Autodesk Inventor part; units mm, degrees
ref_plane "YZ Plane" through (0, 0, 0) normal (1, 0, 0) x (0, 1, 0)
ref_plane "XZ Plane" through (0, 0, 0) normal (0, 1, 0) x (-1, 0, 0)
ref_plane "XY Plane" through (0, 0, 0) normal (0, 0, 1) x (1, 0, 0)
sketch "Sketch1" plane through (0, 0, 0) normal (0, 1, 0) x (-1, 0, 0)
  line L0 (7.415, 10.16) -> (-7.415, 10.16)
  line L1 (-7.415, 10.16) -> (-7.415, -10.16)
  line L2 (-7.415, -10.16) -> (7.415, -10.16)
  line L3 (7.415, -10.16) -> (7.415, 10.16)
  point P0 (0, 0)
  dimension "d0" = 20.32
  dimension "d1" = 10.16
  dimension "d2" = 14.83
  dimension "d3" = 7.415
extrude "Extrusion1" add sketch "Sketch1" along normal blind 3.91
sketch "Sketch2" plane through (0, 0, 0) normal (0, 1, 0) x (-1, 0, 0)
  line L0 (6.465, -5.76) -> (7.465, -5.76)
  line L1 (7.465, -5.76) -> (7.465, -4.24)
  line L2 (7.465, -4.24) -> (6.465, -4.24)
  line L3 (6.465, -4.24) -> (6.465, -5.76)
  line L4 (7.415, -10.16) -> (7.415, 10.16)
  line L5 (-7.415, -10.16) -> (7.415, -10.16)
  circle A0 centre (7.465, -5) radius 0.5724
  point P0 (0, 0)
  dimension "d6" = 1
  dimension "d7" = 1.52
  dimension "d8" = 0.05
  dimension "d9" = 4.4
extrude "Extrusion2" cut sketch "Sketch2" along normal blind 1 contours A0 L4 | L4 A0 L1 | L1 A0
pattern_linear "Rectangular Pattern1" count 6 spacing 2.01 along (0, 0, 1) of "Extrusion2"
mirror "Mirror1" about plane through (0, 0, 0) normal (1, 0, 0) of "Extrusion2", "Rectangular Pattern1"
sketch "Sketch3" plane through (0, 0, 0) normal (0, -1, 0) x (1, 0, 0)
  line L0 (3.695, -10.21) -> (-3.695, -10.21)
  line L1 (-3.695, -10.21) -> (-3.695, -9.21)
  line L2 (-3.695, -9.21) -> (3.695, -9.21)
  line L3 (3.695, -9.21) -> (3.695, -10.21)
  line L4 (7.415, -10.16) -> (-7.415, -10.16)
  ellipse E0 centre (0, -10.21) end of major axis (-3.2399, -10.21) minor radius 0.6001
  point P0 (0, 0)
  dimension "d15" = 0.05
  dimension "d16" = 7.39
  dimension "d17" = 3.695
  dimension "d18" = 1
extrude "Extrusion3" cut sketch "Sketch3" against normal blind 1 contours E0 L4 L0 | L0 E0 | E0 L4
mirror "Mirror2" about plane through (0, 0, 0) normal (0, 0, 1) of "Extrusion3"
properties part number "MC_DK1042"
Part model, mm, in its own coordinate system. A direction names the side the tool comes from. Round coordinates to 2 decimals unless told otherwise and drop trailing zeros. Loops run counter-clockwise (first coordinate to the right, second up) from the corner with the lowest first, then second, coordinate; pieces in that order, holes last. Notation, with made-up numbers: (51.5, -4) -> (90.5, -4) arc R18 cw to (90.5, 4) -> close; hole circle Ø8 at (69.5, 21). An arc over 180 degrees is marked (long way). Use CSV: the item, a comma, the result in double quotes. Start each with the question number.
1) Cut at B-B, the plane z = -1.25. Write the cut outline in (x, y) (3 decimals).
2) Cut at A-A, the plane z = 3.25. Write the cut outline in (x, y) (3 decimals).
3) Pull direction Z, two halves, no side cores. Call faces 4 (the cylindrical face through (-6.893, 0.493, -5.012)), 5 (the flat face through (0, 2, -10.16)), 6 (the flat face through (0, 0, 0)): +Z half, -Z half, draft (parallel to the pull), parting line (faces both ways), or undercut.
4) Wall check: L1, parallel to X at y = 0.95, z = 3.25; L2, parallel to X at y = 0.3, z = 1.5. Give the ranges that are in metal, low to high. Write a range as [from, to].
5) Which spindle directions (+Z, -Z, +X, -X, +Y, -Y) get a long thin tool onto all of the face, cutting with end or side? Do faces 1 (the cylindrical face through (-6.893, 0.493, 1.018)), 2 (the cylindrical face through (6.893, 0.493, -4.988)), 3 (the flat face through (-7.415, 2, 0)). Say none if no direction does.
6) Drop a flat-ended pin along its axis: P1, Ø0.6, axis at x = 0, z = 10, coming from the -Y side. Give the stop position or say it passes through.
Determined:
1,outline,"(-7.415, 1) -> (-6.96, 1) -> (-6.96, 0) -> (6.96, 0) -> (6.96, 1) -> (7.415, 1) -> (7.415, 3.91) -> (-7.415, 3.91) -> close"
2,outline,"(-7.415, 1) -> (-6.933, 1) -> (-6.933, 0) -> (6.933, 0) -> (6.933, 1) -> (7.415, 1) -> (7.415, 3.91) -> (-7.415, 3.91) -> close"
3,face 4,"undercut"
3,face 5,"-Z half"
3,face 6,"draft"
4,L1,"x = [-6.93, 6.93]"
4,L2,"x = [-7.14, 7.14]"
5,face 1,"-X, -Y"
5,face 2,"+X, -Y"
5,face 3,"+Z, -Z, -X, +Y, -Y"
6,P1,"stops at y = 1"
